Autodesk Inventor part; units mm, degrees
ref_plane "YZ Plane" through (0, 0, 0) normal (1, 0, 0) x (0, 1, 0)
ref_plane "XZ Plane" through (0, 0, 0) normal (0, 1, 0) x (-1, 0, 0)
ref_plane "XY Plane" through (0, 0, 0) normal (0, 0, 1) x (1, 0, 0)
sketch "Sketch1" plane through (0, 0, 0) normal (0, 1, 0) x (-1, 0, 0)
  line L0 (3.8, 0) -> (-22.8, 0)
  line L1 (0, -147.7698) -> (0, 222.7404)
  line L2 (-11, -80) -> (-19, -80)
  line L3 (-19, -80) -> (-19, -74)
  line L4 (-19, -74) -> (-14, -74)
  line L5 (-14, -74) -> (-14, 80)
  line L6 (-14, 80) -> (0, 80)
  line L7 (-11, -94.8398) -> (-11, 169.8104) construction
  line L8 (-11, -80) -> (-11, 76)
  line L9 (-11, 76) -> (0, 76)
  dimension "d0" = 38
  dimension "d1" = 28
  dimension "d3" = 22
  dimension "d4" = 160
  dimension "d5" = 6
  dimension "d7" = 4
revolve "Revolution1" add sketch "Sketch1" angle 360 about axis through (0, 0, -10) along (0, 0, 1) contours L8 L2 L3 L4 L5 L0 | L0 L5 L6 L1 L9 L8
fillet "Fillet1" radius 2 4 edges at (-19, 0, -74) (-14, 0, -74) (-14, 0, 80) (-19, 0, -80)
properties part number "Handle bars handles"
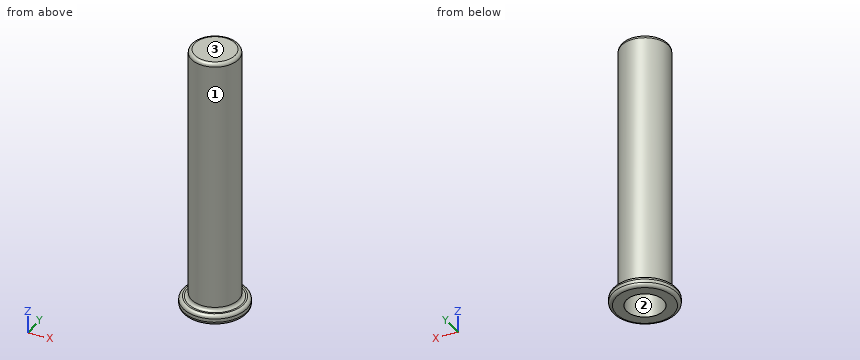
For this review, take the finished solid that the model builds, in its own axes (mm). Face numbers are marked on the shaded views. Round coordinates to 2 decimals unless told otherwise and drop trailing zeros. Write each loop counter-clockwise with the first axis right and the second up, starting at its lowest first coordinate (ties: lowest second). Pieces come first, ordered by that corner, then holes. Notation, with made-up numbers: (77, 41) -> (129, 41) arc R10 cw to (129, 51) -> close; hole circle Ø1 at (-1, 48.25). An arc over 180 degrees is marked (long way). One line per question, with ' | ' between items. Start each with the question number.
(1) Add section C-C, the plane z = 5.5. Write out the cut boundary in (x, y), plus the area to 3 significant figures.
(2) Insertion check: P1, Ø6.5, axis at x = 4, y = 1, coming from the -Z side; P2, Ø12, axis at x = -6.5, y = -5, coming from the -Z side; P3, Ø1, axis at y = 8.5, z = 37.5, coming from the +X side; P4, Ø2, axis at y = 10, z = -47, coming from the +X side. Each pin has a flat end and moves straight along its axis. Give the tip position at first contact, or say it passes through.
(3) Add section A-A, the plane y = 0. Write out the cut boundary in (x, z), plus the area to 3 significant figures.
(4) For line 1 along Y through (x, z) = (0, 29); line 2 along Z through (x, y) = (-6.5, 3); line 3 along X through (y, z) = (-8, -47.5), list the stretches that pass through material, from the lowest coordinate up. Write a range as from..to.
(5) Mouldability with a two-part tool opening along X and no side actions: class the marked faces 1, 2 and 3 as released by +X, released by -X, zero draft, split by the parting line, or undercut.
Answer list:
1) outline: circle Ø28 at (0, 0); hole circle Ø22 at (0, 0) | area: 236 mm²
2) P1: z = 76 | P2: z = -80 | P3: x = 11.49 | P4: x = 10.72
3) outline: (-19, -78) arc R2 ccw to (-17, -80) -> (-11, -80) -> (-11, 76) -> (11, 76) -> (11, -80) -> (17, -80) arc R2 ccw to (19, -78) -> (19, -76) arc R2 ccw to (17, -74) -> (16, -74) arc R2 cw to (14, -72) -> (14, 78) arc R2 ccw to (12, 80) -> (-12, 80) arc R2 ccw to (-14, 78) -> (-14, -72) arc R2 cw to (-16, -74) -> (-17, -74) arc R2 ccw to (-19, -76) -> close | area: 1,100 mm²
4) line 1: -14..-11, 11..14 | line 2: 76..80 | line 3: -11.49..-7.55, 7.55..11.49
5) face 1: split by the parting line | face 2: undercut | face 3: zero draft
